```python
from build123d import *

# Parameters (mm, degrees)
SKETCH1_W            = 8
SKETCH1_H            = 48
BOSS_EXTRUDE1_DEPTH  = 9.6
SKETCH2_R            = 2.4
BOSS_EXTRUDE2_DEPTH  = 1.6
LPATTERN1_COUNT      = 2
LPATTERN1_PITCH      = 8
LPATTERN1_COUNT_DIR2 = 6
LPATTERN1_PITCH_DIR2 = 8
SHELL1_T             = -1.6


with BuildPart() as part:
    # Sketch1 → Boss-Extrude1 (new body)
    with BuildSketch(Plane(origin=(0, 0, 0), x_dir=(1, 0, 0), z_dir=(0, 1, 0))):
        with Locations((4, 24)):
            Rectangle(SKETCH1_W, SKETCH1_H)
    extrude(amount=BOSS_EXTRUDE1_DEPTH)

    # Sketch2 → Boss-Extrude2 (add)
    with BuildSketch(Plane(origin=(0, 9.6, 0), x_dir=(1, 0, 0), z_dir=(0, 1, 0))):
        with Locations(Location((4, 4, 0), (0, 0, 90))):
            Circle(SKETCH2_R)
    boss_extrude2 = extrude(amount=BOSS_EXTRUDE2_DEPTH)

    # LPattern1: Boss-Extrude2 2 × 6, 6 skipped
    with Locations(*[(i * LPATTERN1_PITCH, 0, -j * LPATTERN1_PITCH_DIR2) for i in range(LPATTERN1_COUNT) for j in range(LPATTERN1_COUNT_DIR2) if (i, j) not in ((0, 0), (1, 0), (1, 1), (1, 2), (1, 3), (1, 4), (1, 5))]):
        add(boss_extrude2)

    # Shell1
    shell1_openings = [part.faces().sort_by_distance(p)[0] for p in [
        (4, 0, -24),
    ]]
    offset(amount=SHELL1_T, openings=shell1_openings, kind=Kind.INTERSECTION)


solid = part.part
```
Read the model definition and answer for the solid it produces. Units are mm, in the model's axes. A direction names the side the tool comes from. Give positions to 0.01 mm unless a question says otherwise; leave off trailing zeros. Write each loop counter-clockwise with the first axis right and the second up, starting at its lowest first coordinate (ties: lowest second). Pieces come first, ordered by that corner, then holes. Notation, with made-up numbers: M 46,20.5 L 65,20.5 A26 ccw 65,47.5 Z; hole C 69,20.5 d7. An arc over 180 degrees is marked long. Put each result on its own line as item: value. Start each with the question number.
1. Which of the six approach directions +Z, -Z, +X, -X, +Y, -Y give full straight-line access (tool end or side, diameter ignored) to faces 1 (the flat face through (4, 11.2, -4)), 2 (the flat face through (4, 4, -46.4)), 3 (the cylindrical face through (3.894, 10.389, -17.602))?
2. Consider line 1 along X through (y, z) = (5.5, -37.5); line 2 along X through (y, z) = (8.4, -28); line 3 along Z through (x, y) = (3, 10.25). Determine where each line is inside the solid, lowest interval first.
3. Each of these flat-tipped pins is pushed along its axis until it touches: pin 1 Ø1.3 at (x, z) = (4, -28) entering from -Y; pin 2 Ø3 at (x, z) = (1.5, -23.5) entering from -Y; pin 3 Ø2.5 at (x, z) = (4, -36) entering from -Y. Where does it stop, or does it pass through?
4. The part is cut by section B-B, the plane z = -16. Give the vertices of the cut face in (x, y).
5. The part is cut by section C-C, the plane y = 10. Give the vertices of the cut face in (x, z), and give its area (3 significant figures).
6. For a pull along Z with two mould halves and no side action, classify faces 4 (the flat face through (4, 11.2, -20)), 5 (the flat face through (4, 5, 0)), 6 (the flat face through (6.4, 4, -24)) as released by +Z, released by -Z, zero draft, split by the parting line, or undercut.
7. The part is cut by section A-A, the plane y = 6.5. Give the vertices of the cut face in (x, z), and give its area (3 significant figures).
8. The part is cut by section D-D, the plane z = -44. Give the vertices of the cut face in (x, y), and give its area (3 significant figures).
Final values:
1. face 1: +Z, -Z, +X, -X, +Y
1. face 2: -Y
1. face 3: +Y
2. line 1: x = 0 to 1.6, 6.4 to 8
2. line 2: x = 0 to 3.2, 4.8 to 8
2. line 3: z = -46.18 to -41.82, -38.18 to -33.82, -30.18 to -25.82, -22.18 to -17.82, -14.18 to -9.82, -6.18 to -1.82
3. pin 1: stops at y = 9.6
3. pin 2: stops at y = 0
3. pin 3: stops at y = 8
4. outline: M 0,0 L 1.6,0 L 1.6,8 L 6.4,8 L 6.4,0 L 8,0 L 8,9.6 L 0,9.6 Z
5. outline: C 4,-44 d4.8; C 4,-36 d4.8; C 4,-28 d4.8; C 4,-20 d4.8; C 4,-12 d4.8; C 4,-4 d4.8
5. area: 109 mm²
6. face 4: zero draft
6. face 5: released by +Z
6. face 6: undercut
7. outline: M 0,-48 L 8,-48 L 8,0 L 0,0 Z; hole M 1.6,-46.4 L 6.4,-46.4 L 6.4,-1.6 L 1.6,-1.6 Z
7. area: 169 mm²
8. outline: M 0,0 L 1.6,0 L 1.6,8 L 3.2,8 L 3.2,9.6 L 4.8,9.6 L 4.8,8 L 6.4,8 L 6.4,0 L 8,0 L 8,9.6 L 6.4,9.6 L 6.4,11.2 L 1.6,11.2 L 1.6,9.6 L 0,9.6 Z
8. area: 43.5 mm²
